The listing builds one solid part. Answer for the finished solid, in the listing's coordinates (mm). Face numbers are marked on the shaded views. A direction names the side the tool comes from. Give positions to 0.01 mm unless a question says otherwise; leave off trailing zeros. One line per question, with ' | ' between items. Start each with the question number.
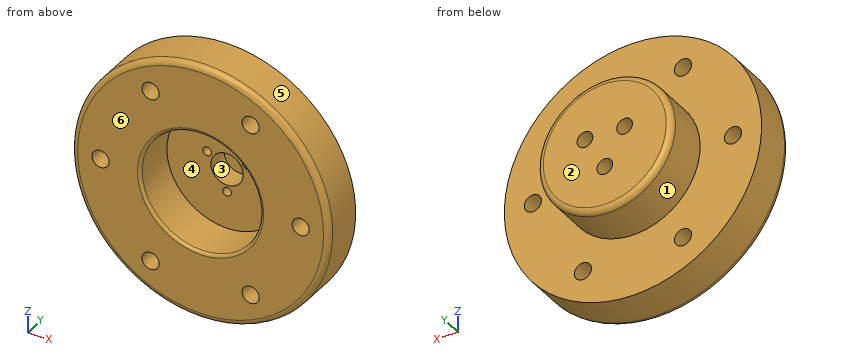
from build123d import *

# Parameters (mm, degrees)
SKETCH1_R           = 23.5
BOSS_EXTRUDE1_DEPTH = 14
SKETCH2_R           = 25
SKETCH2_R_2         = 21.05
BOSS_EXTRUDE2_DEPTH = 15
SKETCH3_R           = 5.65
SKETCH3_R_2         = 1.5
CUT_EXTRUDE1_DEPTH  = 7.5
SKETCH4_R           = 23.5
SKETCH4_R_2         = 1.517776155
SKETCH4_R_3         = 1.5
BOSS_EXTRUDE3_DEPTH = 2
SKETCH5_R           = 2.75
CUT_EXTRUDE2_DEPTH  = 6
SKETCH6_R           = 1.5
CUT_EXTRUDE3_DEPTH  = 42.907636536
CHAMFER1_SIZE       = 1.3
BOSS_EXTRUDE5_START = -15
SKETCH7_R           = 45
SKETCH7_R_2         = 3
SKETCH7_R_3         = 23.5
BOSS_EXTRUDE5_DEPTH = 15
FILLET1_R           = 2
FILLET2_R           = 1


# Some blends are built 0.0001 mm under size
with BuildPart() as part:
    # Sketch1 → Boss-Extrude1 (new body)
    with BuildSketch(Plane(origin=(0, 0, 0), x_dir=(1, 0, 0), z_dir=(0, 1, 0))):
        with Locations(Location((0, 0, 0), (0, 0, 270))):
            Circle(SKETCH1_R)
    extrude(amount=BOSS_EXTRUDE1_DEPTH)

    # Sketch2 → Boss-Extrude2 (add)
    with BuildSketch(Plane.XZ):
        with Locations(Location((0, 0, 0), (0, 0, 270))):
            Circle(SKETCH2_R)
        with Locations(Location((0, 0, 0), (0, 0, 270))):
            Circle(SKETCH2_R_2, mode=Mode.SUBTRACT)
    extrude(amount=BOSS_EXTRUDE2_DEPTH)

    # Sketch3 → Cut-Extrude1 (cut)
    with BuildSketch(Plane(origin=(0, 0, 0), x_dir=(-1, 0, 0), z_dir=(0, -1, 0))):
        with Locations(Location((0, 0, 0), (0, 0, 90))):
            Circle(SKETCH3_R)
        with Locations(Location((0, 8, 0), (0, 0, 90))):
            Circle(SKETCH3_R_2)
        with Locations(Location((6.92820323, -4, 0), (0, 0, 90))):
            Circle(SKETCH3_R_2)
        with Locations(Location((-6.92820323, -4, 0), (0, 0, 90))):
            Circle(SKETCH3_R_2)
    extrude(amount=-CUT_EXTRUDE1_DEPTH, mode=Mode.SUBTRACT)

    # Sketch4 → Boss-Extrude3 (add)
    with BuildSketch(Plane(origin=(0, 14, 0), x_dir=(1, 0, 0), z_dir=(0, 1, 0))):
        with Locations(Location((0, 0, 0), (0, 0, 90))):
            Circle(SKETCH4_R)
        with Locations(Location((0, 8, 0), (0, 0, 270))):
            Circle(SKETCH4_R_2, mode=Mode.SUBTRACT)
        with Locations(Location((6.92820323, -4, 0), (0, 0, 90))):
            Circle(SKETCH4_R_3, mode=Mode.SUBTRACT)
        with Locations(Location((-6.92820323, -4, 0), (0, 0, 90))):
            Circle(SKETCH4_R_3, mode=Mode.SUBTRACT)
    extrude(amount=BOSS_EXTRUDE3_DEPTH)

    # Sketch5 → Cut-Extrude2 (cut)
    with BuildSketch(Plane(origin=(0, 16, 0), x_dir=(1, 0, 0), z_dir=(0, 1, 0))):
        with Locations(Location((0, 8, 0), (0, 0, 270))):
            Circle(SKETCH5_R)
        with Locations(Location((6.92820323, -4, 0), (0, 0, 270))):
            Circle(SKETCH5_R)
        with Locations(Location((-6.92820323, -4, 0), (0, 0, 270))):
            Circle(SKETCH5_R)
    extrude(amount=-CUT_EXTRUDE2_DEPTH, mode=Mode.SUBTRACT)

    # Sketch6 → Cut-Extrude3 (cut, through all)
    with BuildSketch(Plane.XZ.offset(-7.5)):
        with Locations(Location((-6.92820323, 4, 0), (0, 0, 270))):
            Circle(SKETCH6_R)
        with Locations(Location((0, -8, 0), (0, 0, 270))):
            Circle(SKETCH6_R)
        with Locations(Location((6.92820323, 4, 0), (0, 0, 270))):
            Circle(SKETCH6_R)
    extrude(amount=-CUT_EXTRUDE3_DEPTH, mode=Mode.SUBTRACT)

    # Chamfer1
    # the kernel refuses this chamfer: 1.3 mm, written as the material it takes off along each edge
    with BuildSketch(Plane(origin=(0, 10, -8), x_dir=(0, 0, -1), z_dir=(-1, 0, 0))) as chamfer1_piece_1_section:
        Polygon((1.5 + CHAMFER1_SIZE, 0), (1.5, CHAMFER1_SIZE), (1.5, 0), align=None)
    chamfer1_piece_1 = revolve(axis=Axis((0, 10, -8), (0, -1, 0)), mode=Mode.PRIVATE)
    chamfer1_piece_1 = chamfer1_piece_1 & Plane(origin=(0, 9.322421141, -8), x_dir=(0, 0, 1), z_dir=(0, 1, 0)) * Cylinder(2.75, 12, mode=Mode.PRIVATE)
    add(chamfer1_piece_1, mode=Mode.SUBTRACT)
    with BuildSketch(Plane(origin=(-6.92820323, 10, 4), x_dir=(0, 0, -1), z_dir=(-1, 0, 0))) as chamfer1_piece_2_section:
        Polygon((1.5 + CHAMFER1_SIZE, 0), (1.5, CHAMFER1_SIZE), (1.5, 0), align=None)
    chamfer1_piece_2 = revolve(axis=Axis((-6.92820323, 10, 4), (0, -1, 0)), mode=Mode.PRIVATE)
    chamfer1_piece_2 = chamfer1_piece_2 & Plane(origin=(-6.92820323, 9.322421141, 4), x_dir=(0, 0, 1), z_dir=(0, 1, 0)) * Cylinder(2.75, 12, mode=Mode.PRIVATE)
    add(chamfer1_piece_2, mode=Mode.SUBTRACT)
    with BuildSketch(Plane(origin=(6.92820323, 10, 4), x_dir=(0, 0, -1), z_dir=(-1, 0, 0))) as chamfer1_piece_3_section:
        Polygon((1.5 + CHAMFER1_SIZE, 0), (1.5, CHAMFER1_SIZE), (1.5, 0), align=None)
    chamfer1_piece_3 = revolve(axis=Axis((6.92820323, 10, 4), (0, -1, 0)), mode=Mode.PRIVATE)
    chamfer1_piece_3 = chamfer1_piece_3 & Plane(origin=(6.92820323, 9.322421141, 4), x_dir=(0, 0, 1), z_dir=(0, 1, 0)) * Cylinder(2.75, 12, mode=Mode.PRIVATE)
    add(chamfer1_piece_3, mode=Mode.SUBTRACT)

    # Sketch7 → Boss-Extrude5 (add)
    with BuildSketch(Plane(origin=(0, 0, 0), x_dir=(1, 0, 0), z_dir=(0, 1, 0)).offset(BOSS_EXTRUDE5_START)):
        with Locations(Location((0, 0, 0), (0, 0, 270))):
            Circle(SKETCH7_R)
        with Locations(Location((-35, 0, 0), (0, 0, 270))):
            Circle(SKETCH7_R_2, mode=Mode.SUBTRACT)
        with Locations(Location((-17.4995, 30.311755158, 0), (0, 0, 270))):
            Circle(SKETCH7_R_2, mode=Mode.SUBTRACT)
        with Locations(Location((17.5015, 30.311755158, 0), (0, 0, 270))):
            Circle(SKETCH7_R_2, mode=Mode.SUBTRACT)
        with Locations(Location((35.002, 0, 0), (0, 0, 270))):
            Circle(SKETCH7_R_2, mode=Mode.SUBTRACT)
        with Locations(Location((17.5015, -30.311755158, 0), (0, 0, 270))):
            Circle(SKETCH7_R_2, mode=Mode.SUBTRACT)
        with Locations(Location((-17.4995, -30.311755158, 0), (0, 0, 270))):
            Circle(SKETCH7_R_2, mode=Mode.SUBTRACT)
        with Locations(Location((0, 0, 0), (0, 0, 90))):
            Circle(SKETCH7_R_3, mode=Mode.SUBTRACT)
    extrude(amount=BOSS_EXTRUDE5_DEPTH)

    # Fillet1
    fillet1_edges = [part.edges().sort_by_distance(p)[0] for p in [
        (0, 16, 23.5),
        (0, -15, -45),
    ]]
    fillet(fillet1_edges, radius=FILLET1_R - 0.0001)  # a hair under: the kernel refuses the full size

    # Fillet2
    fillet2_edges = [part.edges().sort_by_distance(p)[0] for p in [
        (0, -15, 21.05),
    ]]
    fillet(fillet2_edges, radius=FILLET2_R)


solid = part.part
1. Determine the mould class of the marked faces 4, 5 and 6 for opening direction X: released by +X, released by -X, zero draft, split by the parting line, or undercut.
2. For the marked faces 1, 2 and 3, determine the directions among +Z, -Z, +X, -X, +Y, -Y from which every point of the face is accessible in a straight line to the end or side of a thin tool.
3. Each of these flat-tipped pins is pushed along its axis until it touches: pin 1 Ø21 at (x, z) = (4.5, -6.5) entering from -Y; pin 2 Ø9.5 at (x, z) = (17.5, -30.31) entering from +Y; pin 3 Ø3 at (x, y) = (30.5, -4) entering from -Z. Where does it stop, or does it pass through?
4. Straight lines are drawn through the part: L1, parallel to X at y = 3, z = 0; L2, parallel to X at y = 6.75, z = 4; L3, parallel to Z at x = 0, y = 13.75. For each, find the intervals that lie inside material, in ascending order.
5. The part is cut by section B-B (z = 0). Count the separate pieces of the cut face and the enclosed holes in it, plus the area to 3 significant figures.
Check sheet entries:
1) face 4: undercut | face 5: split by the parting line | face 6: zero draft
2) face 1: +Y | face 2: +Z, -Z, +X, -X, +Y | face 3: -Y
3) pin 1: stops at y = 0 | pin 2: stops at y = 0 | pin 3: stops at z = -34.41
4) L1: x = -23.5 to -5.65, 5.65 to 23.5 | L2: x = -23.16 to -8.43, -5.43 to -3.99, 3.99 to 5.43, 8.43 to 23.16 | L3: z = -23.5 to -10.75, -5.25 to 23.5
5) separate pieces: 3 | enclosed holes: 0 | area: 1,200 mm^2
